Geometry: final body of the model. Coordinates: model frame, mm. A direction names the side the tool comes from. Give positions to 0.01 mm unless a question says otherwise; leave off trailing zeros. Loops run counter-clockwise (first coordinate to the right, second up) from the corner with the lowest first, then second, coordinate; pieces in that order, holes last. Notation, with made-up numbers: (79.25, -22) -> (83.25, -22) arc R22 cw to (83.25, -11) -> close; hole circle Ø9 at (88.25, 79.5). An arc over 180 degrees is marked (long way). Answer in a Markdown table with one row per item. Add a question column.
from build123d import *

# Parameters (mm, degrees)
BOSS_EXTRUDE1_DEPTH                       = 150
BOSS_EXTRUDE1_DRAFT                       = -2.8
CUT_EXTRUDE1_DEPTH                        = 157.704023919
CUT_EXTRUDE1_DRAFT                        = -2.8
CUT_EXTRUDE1_PROFILE_2_DEPTH              = 157.704023919
CUT_EXTRUDE1_PROFILE_2_DRAFT              = -2.8
SKETCH4_W                                 = 86.570961738
SKETCH4_H                                 = 17.749989686
CUT_EXTRUDE2_DEPTH                        = 157.704023919
BOSS_EXTRUDE2_DEPTH                       = 3.8
BOSS_EXTRUDE3_DEPTH                       = 3.8
CBORE_FOR_M4_SBHCS1_D                     = 4.2
CBORE_FOR_M4_SBHCS1_CBORE_D               = 8
CBORE_FOR_M4_SBHCS1_CBORE_DEPTH           = 2.2
CBORE_FOR_M4_SBHCS1_ON_FACE_2_D           = 4.2
CBORE_FOR_M4_SBHCS1_ON_FACE_2_CBORE_D     = 8
CBORE_FOR_M4_SBHCS1_ON_FACE_2_CBORE_DEPTH = 2.2
CBORE_FOR_M4_SBHCS1_ON_FACE_3_D           = 4.2
CBORE_FOR_M4_SBHCS1_ON_FACE_3_CBORE_D     = 8
CBORE_FOR_M4_SBHCS1_ON_FACE_3_CBORE_DEPTH = 2.2
CBORE_FOR_M4_SBHCS1_ON_FACE_4_D           = 4.2
CBORE_FOR_M4_SBHCS1_ON_FACE_4_CBORE_D     = 8
CBORE_FOR_M4_SBHCS1_ON_FACE_4_CBORE_DEPTH = 2.2
CBORE_FOR_M4_SBHCS1_ON_FACE_5_D           = 4.2
CBORE_FOR_M4_SBHCS1_ON_FACE_5_CBORE_D     = 8
CBORE_FOR_M4_SBHCS1_ON_FACE_5_CBORE_DEPTH = 2.2


with BuildPart() as part:
    # Sketch1 → Boss-Extrude1 (with draft: the straight prism first)
    with BuildSketch(Plane.XY):
        with BuildLine():
            Line((-7.5, 0), (7.5, 0))
            ThreePointArc((7.5, 0), (22.10898696, 5.783678888), (28.8, 20))
            Line((28.8, 20), (-28.8, 20))
            ThreePointArc((-28.8, 20), (-22.10898696, 5.783678888), (-7.5, 0))
        make_face()
    extrude(amount=BOSS_EXTRUDE1_DEPTH)
    # Boss-Extrude1: the draft: its side faces are tilted about the plane it starts from
    boss_extrude1_sides = [part.faces().sort_by_distance(p)[0] for p in [
        (0, 0, 75),
        (22.10898696, 5.783678888, 75),
        (0, 20, 75),
        (-22.10898696, 5.783678888, 75),
    ]]
    draft(boss_extrude1_sides, Plane.XY, BOSS_EXTRUDE1_DRAFT)


with BuildPart() as cut_extrude1_tool:
    # Sketch1_3 → Cut-Extrude1 (with draft: the straight prism first)
    with BuildSketch(Plane.XY):
        with BuildLine():
            ThreePointArc((-24.271636772, 16.2), (-17.92889975, 7.236627537), (-7.5, 3.8))
            Line((-7.5, 3.8), (7.5, 3.8))
            ThreePointArc((7.5, 3.8), (17.92889975, 7.236627537), (24.271636772, 16.2))
            Line((24.271636772, 16.2), (-24.271636772, 16.2))
        make_face()
    extrude(amount=CUT_EXTRUDE1_DEPTH)
    # Cut-Extrude1: the draft: its side faces are tilted about the plane it starts from
    cut_extrude1_sides = [cut_extrude1_tool.faces().sort_by_distance(p)[0] for p in [
        (17.92889975, 7.236627537, 78.85201196),
        (0, 16.2, 78.85201196),
        (-17.92889975, 7.236627537, 78.85201196),
        (0, 3.8, 78.85201196),
    ]]
    draft(cut_extrude1_sides, Plane.XY, CUT_EXTRUDE1_DRAFT)


with BuildPart() as part_1:
    add(part.part)

    # Cut-Extrude1: cut by cut_extrude1_tool
    add(cut_extrude1_tool.part, mode=Mode.SUBTRACT)


with BuildPart() as cut_extrude1_profile_2_tool:
    # Sketch1_3 → Cut-Extrude1 profile 2 (with draft: the straight prism first)
    with BuildSketch(Plane.XY):
        with BuildLine():
            Line((24.990823308, 20), (-24.990823308, 20))
            ThreePointArc((-24.990823308, 20), (-24.736271136, 18.080119963), (-24.271636772, 16.2))
            Line((-24.271636772, 16.2), (24.271636772, 16.2))
            ThreePointArc((24.271636772, 16.2), (24.736271136, 18.080119963), (24.990823308, 20))
        make_face()
    extrude(amount=CUT_EXTRUDE1_PROFILE_2_DEPTH)
    # Cut-Extrude1 profile 2: the draft: its side faces are tilted about the plane it starts from
    cut_extrude1_profile_2_sides = [cut_extrude1_profile_2_tool.faces().sort_by_distance(p)[0] for p in [
        (0, 20, 78.85201196),
        (-24.736271136, 18.080119963, 78.85201196),
        (0, 16.2, 78.85201196),
        (24.736271136, 18.080119963, 78.85201196),
    ]]
    draft(cut_extrude1_profile_2_sides, Plane.XY, CUT_EXTRUDE1_PROFILE_2_DRAFT)


with BuildPart() as part_2:
    add(part_1.part)

    # Cut-Extrude1 profile 2: cut by cut_extrude1_profile_2_tool
    add(cut_extrude1_profile_2_tool.part, mode=Mode.SUBTRACT)

    # Sketch4 → Cut-Extrude2 (cut, through all)
    with BuildSketch(Plane(origin=(0, 0, 0), x_dir=(-1, 0, 0), z_dir=(0, 0, -1))):
        with Locations((0, 28.874994843)):
            Rectangle(SKETCH4_W, SKETCH4_H)
    extrude(amount=-CUT_EXTRUDE2_DEPTH, mode=Mode.SUBTRACT)

    # Sketch5 → Boss-Extrude2 (add)
    with BuildSketch(Plane(origin=(28.773423739, 0, -1.407255195), x_dir=(-0.04884976979561336, 0, -0.9988061373414341), z_dir=(0.9988061373414341, 0, -0.04884976979561336))):
        Polygon((-149.586695466, 20), (-147.336695466, 27.5), (-119.836695466, 27.5), (-117.586695466, 20), (-123.586695466, 20), (-123.586695466, 23), (-143.586695466, 23), (-143.586695466, 20), align=None)
        Polygon((-9.40687337, 23), (-9.40687337, 20), (-3.40687337, 20), (-5.65687337, 27.5), (-33.15687337, 27.5), (-35.40687337, 20), (-29.40687337, 20), (-29.40687337, 23), align=None)
    extrude(amount=-BOSS_EXTRUDE2_DEPTH)

    # Sketch6 → Boss-Extrude3 (add)
    with BuildSketch(Plane(origin=(-28.773423739, 0, -1.407255195), x_dir=(-0.04884976979561336, 0, 0.9988061373414341), z_dir=(-0.9988061373414341, 0, -0.04884976979561336))):
        Polygon((149.586695466, 20), (147.336695466, 27.5), (119.836695466, 27.5), (117.586695466, 20), (123.586695466, 20), (123.586695466, 23), (143.586695466, 23), (143.586695466, 20), align=None)
        Polygon((9.40687337, 23), (9.40687337, 20), (3.40687337, 20), (5.65687337, 27.5), (33.15687337, 27.5), (35.40687337, 20), (29.40687337, 20), (29.40687337, 23), align=None)
    extrude(amount=-BOSS_EXTRUDE3_DEPTH)

    # CBORE for M4 SBHCS1 (through all)
    with Locations(Plane(origin=(0, -2.017501828, 118.947470043), x_dir=(0, -0.048849769796, 0.998806137341), z_dir=(0, 0.998806137341, 0.048849769796))):
        with Locations((0, 0)):
            CounterBoreHole(CBORE_FOR_M4_SBHCS1_D / 2, CBORE_FOR_M4_SBHCS1_CBORE_D / 2, CBORE_FOR_M4_SBHCS1_CBORE_DEPTH)

    # CBORE for M4 SBHCS1 on face 2 (through all)
    with Locations(Plane(origin=(0, -0.942806892, 96.973735022), x_dir=(0, -0.048850006152, 0.998806125782), z_dir=(0, 0.998806125782, 0.048850006152))):
        with Locations((0, 0)):
            CounterBoreHole(CBORE_FOR_M4_SBHCS1_ON_FACE_2_D / 2, CBORE_FOR_M4_SBHCS1_ON_FACE_2_CBORE_D / 2, CBORE_FOR_M4_SBHCS1_ON_FACE_2_CBORE_DEPTH)

    # CBORE for M4 SBHCS1 on face 3 (through all)
    with Locations(Plane(origin=(0, 0.131888043, 75), x_dir=(0, -0.048850006152, 0.998806125782), z_dir=(0, 0.998806125782, 0.048850006152))):
        with Locations((0, 0)):
            CounterBoreHole(CBORE_FOR_M4_SBHCS1_ON_FACE_3_D / 2, CBORE_FOR_M4_SBHCS1_ON_FACE_3_CBORE_D / 2, CBORE_FOR_M4_SBHCS1_ON_FACE_3_CBORE_DEPTH)

    # CBORE for M4 SBHCS1 on face 4 (through all)
    with Locations(Plane(origin=(0, 1.206582979, 53.026264978), x_dir=(0, -0.048850006152, 0.998806125782), z_dir=(0, 0.998806125782, 0.048850006152))):
        with Locations((0, 0)):
            CounterBoreHole(CBORE_FOR_M4_SBHCS1_ON_FACE_4_D / 2, CBORE_FOR_M4_SBHCS1_ON_FACE_4_CBORE_D / 2, CBORE_FOR_M4_SBHCS1_ON_FACE_4_CBORE_DEPTH)

    # CBORE for M4 SBHCS1 on face 5 (through all)
    with Locations(Plane(origin=(0, 2.281277914, 31.052529957), x_dir=(0, -0.048850006152, 0.998806125782), z_dir=(0, 0.998806125782, 0.048850006152))):
        with Locations((0, 0)):
            CounterBoreHole(CBORE_FOR_M4_SBHCS1_ON_FACE_5_D / 2, CBORE_FOR_M4_SBHCS1_ON_FACE_5_CBORE_D / 2, CBORE_FOR_M4_SBHCS1_ON_FACE_5_CBORE_DEPTH)


solid = part_2.part
(1) Pin query (flat end, axial travel): pin 1 Ø2 at (x, z) = (8.5, 35.5) entering from -Y; pin 2 Ø4 at (x, z) = (-33, 129.5) entering from -Y; pin 3 Ø3.5 at (x, z) = (32.5, 38.5) entering from +Y; pin 4 Ø3.5 at (x, z) = (-29, 84.5) entering from +Y. Return the tip coordinate at first contact, or that it passes through.
(2) Draft query along Y for faces 1 (the flat face through (34.155, 23.698, 146.984)), 2 (the flat face through (31, 20, 80)), 3 (the flat face through (-29.732, 24.636, 18.2)), 4 (the flat face through (-31, 20, 80)). Return one class per face: +Y half, -Y half, draft (parallel to the pull), parting line (faces both ways), or undercut.
(3) Cut plane B-B on z = 44. Return the cut outline in (x, y), then the cut area to 3 significant figures.
(4) Cut plane D-D on z = 65.5. Return the cut outline in (x, y).
(5) Cut plane C-C on x = 6. Return the cut outline in (y, z).
(6) Reachability of faces 5 (the flat face through (-28.58, 23.8, 32.91)), 6 (the flat face through (-32.7, 23.8, 117.27)), 7 (the flat face through (-5.105, 0.183, 73.95)), 8 (the flat face through (28.339, 21.479, 28.056)), 9 (the flat face through (0, -4, 150)) from +Z, -Z, +X, -X, +Y, -Y: full face, straight path, thin tool, end or side. Return the list, or none.
(7) Material intervals for line 1 along X through (y, z) = (13, 8); line 2 along X through (y, z) = (1, 131.5); line 3 along Y through (x, z) = (0, 66), sorted ascending. Write a range as from..to.
(8) Cut plane A-A on y = 25.5. Return the cut outline in (x, z), then the cut area to 3 significant figures.
Answer list:
| question | item | result |
|---|---|---|
| 1 | pin 1 | stops at y = -1.77 |
| 1 | pin 2 | stops at y = 6.72 |
| 1 | pin 3 | passes through |
| 1 | pin 4 | stops at y = 20 |
| 2 | face 1 | +Y half |
| 2 | face 2 | undercut |
| 2 | face 3 | draft |
| 2 | face 4 | undercut |
| 3 | outline | (-30.96, 20) arc R23.49 ccw to (-7.5, -2.15) -> (7.5, -2.15) arc R23.49 ccw to (30.96, 20) -> (27.15, 20) arc R19.69 cw to (7.5, 1.65) -> (-7.5, 1.65) arc R19.69 cw to (-27.15, 20) -> close |
| 3 | area | 305 mm² |
| 4 | outline | (-32.01, 20) arc R24.55 ccw to (-7.5, -3.2) -> (7.5, -3.2) arc R24.55 ccw to (32.01, 20) -> (28.2, 20) arc R20.75 cw to (7.5, 0.6) -> (-7.5, 0.6) arc R20.75 cw to (-28.2, 20) -> close |
| 5 | outline | (-7.34, 150) -> (0, 0) -> (3.8, 0) -> (-3.54, 150) -> close |
| 6 | face 5 | +Z, -X, +Y |
| 6 | face 6 | -Z, +Y |
| 6 | face 7 | +Z, +Y |
| 6 | face 8 | none |
| 6 | face 9 | +Z, +X, -X, +Y, -Y |
| 7 | line 1 | x = -27.57..-23.38, 23.38..27.57 |
| 7 | line 2 | x = -26.41..-20.19, 20.19..26.41 |
| 7 | line 3 | y = -3.23..0.57 |
| 8 | outline | (-36, 146.35) -> (-34.6, 117.69) -> (-30.8, 117.87) -> (-32.2, 146.54) -> close; (-30.42, 32.31) -> (-29.02, 3.64) -> (-25.22, 3.83) -> (-26.63, 32.49) -> close; (25.22, 3.83) -> (29.02, 3.64) -> (30.42, 32.31) -> (26.63, 32.49) -> close; (30.8, 117.87) -> (34.6, 117.69) -> (36, 146.35) -> (32.2, 146.54) -> close |
| 8 | area | 436 mm² |
